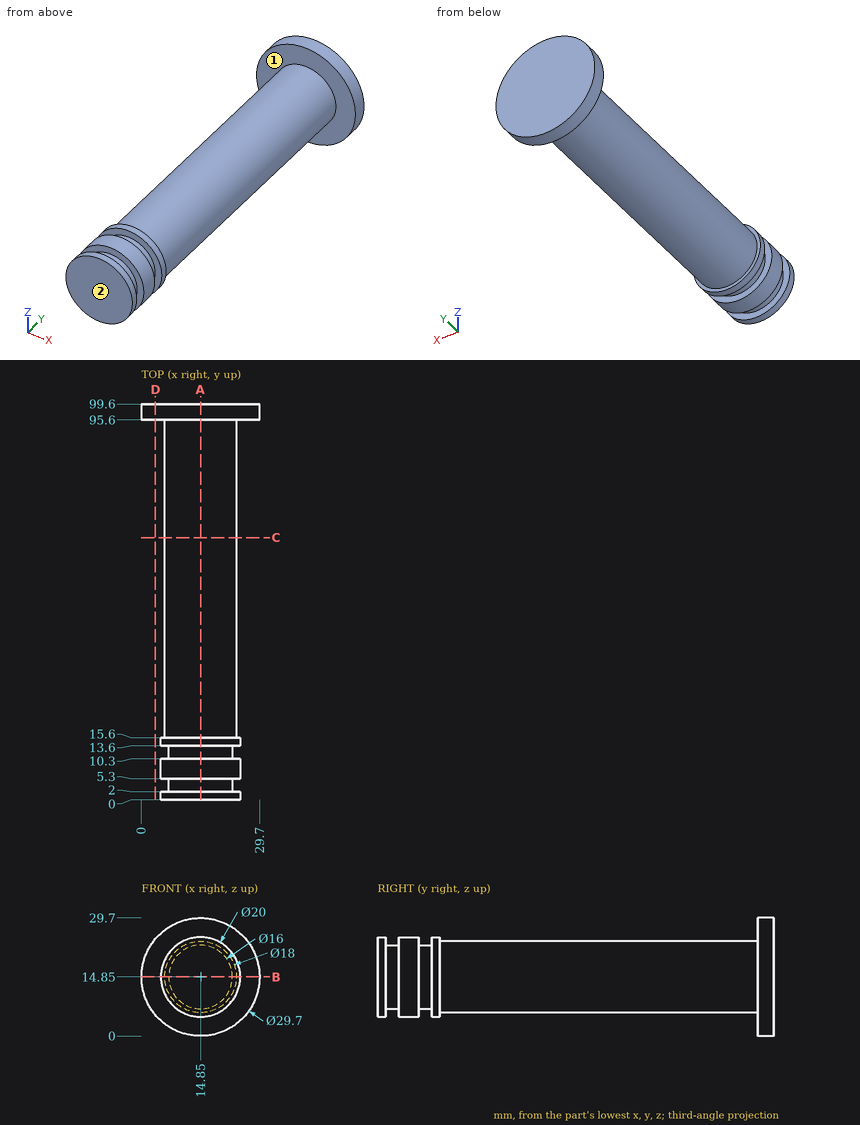
Input: dimensioned drawing with shaded views. Units: mm. Origin: part minimum x, y, z. A direction names the side the tool comes from. Coordinates: 2 decimals unless noted, no trailing zeros. Order: outer loops, then holes, each group sorted by start corner. A loop starts at its lowest first (then second) coordinate and runs counter-clockwise, first axis right, second up. Notation, with made-up numbers: M 30.5,76.25 L 81.5,76.25 A17 ccw 81.5,97.25 Z; hole C 43.5,-28.75 d8. An arc over 180 degrees is marked long. Write each question's results on one line, items separated by ' | '. Start each with the question number.
Item 1: Cut plane A-A (x = 14.85). Return loops of the section in (y, z).
Item 2: Cut plane C-C (y = 66). Return loops of the section in (x, z), and give its area (3 significant figures).
Item 3: Line query: probe 1 along Y at (x, z) = (19.5, 21.75); probe 2 along Y at (x, z) = (15, 3.75); probe 3 along Z at (x, y) = (14.75, 45.5). Output: solid intervals per line, ascending.
Item 4: Cut plane B-B (z = 14.85). Return loops of the section in (x, y), and give its area (3 significant figures).
Item 5: Set-up query: the marked faces 1 and 2. Return all of +Z, -Z, +X, -X, +Y, -Y with unobstructed straight access to the full face (end or side cutting, diameter ignored); none if empty.
Item 6: Cut plane D-D (x = 3.5). Return loops of the section in (y, z).
Item 7: First-contact query: pin 1 Ø12 at (x, y) = (20, 49) entering from +Z; pin 2 Ø12 at (y, z) = (34.5, 26.5) entering from +X; pin 3 Ø4 at (y, z) = (44.5, 14) entering from +X. Flat tips, straight axial feed; report the tip coordinate or a pass-through.
Checked values:
1) outline: M 0,4.85 L 2,4.85 L 2,6.85 L 5.3,6.85 L 5.3,4.85 L 10.3,4.85 L 10.3,6.85 L 13.6,6.85 L 13.6,4.85 L 15.6,4.85 L 15.6,5.85 L 95.6,5.85 L 95.6,0 L 99.6,0 L 99.6,29.7 L 95.6,29.7 L 95.6,23.85 L 15.6,23.85 L 15.6,24.85 L 13.6,24.85 L 13.6,22.85 L 10.3,22.85 L 10.3,24.85 L 5.3,24.85 L 5.3,22.85 L 2,22.85 L 2,24.85 L 0,24.85 Z
2) outline: C 14.85,14.85 d18 | area: 254 mm2
3) probe 1: y = 0 to 2, 5.3 to 10.3, 13.6 to 99.6 | probe 2: y = 95.6 to 99.6 | probe 3: z = 5.85 to 23.85
4) outline: M 0,95.6 L 5.85,95.6 L 5.85,15.6 L 4.85,15.6 L 4.85,13.6 L 6.85,13.6 L 6.85,10.3 L 4.85,10.3 L 4.85,5.3 L 6.85,5.3 L 6.85,2 L 4.85,2 L 4.85,0 L 24.85,0 L 24.85,2 L 22.85,2 L 22.85,5.3 L 24.85,5.3 L 24.85,10.3 L 22.85,10.3 L 22.85,13.6 L 24.85,13.6 L 24.85,15.6 L 23.85,15.6 L 23.85,95.6 L 29.7,95.6 L 29.7,99.6 L 0,99.6 Z | area: 1,840 mm2
5) face 1: none | face 2: +Z, -Z, +X, -X, -Y
6) outline: M 95.6,5.27 L 99.6,5.27 L 99.6,24.43 L 95.6,24.43 Z
7) pin 1: stops at z = 23.85 | pin 2: stops at x = 21.86 | pin 3: stops at x = 23.85
